from build123d import *
from build123d.topology import SkipClean

# Parameters (mm, degrees)
ESQUISSE1_R             = 1.2
BOSS_EXTRU_1_DEPTH      = 12
BOSS_EXTRU_2_DEPTH      = 12
ESQUISSE3_OUTSIDE_W     = 37.484
ESQUISSE3_OUTSIDE_H     = 73.419
ENL_V_MAT_EXTRU_1_DEPTH = 170.970209289
CONG_2_R                = 3
CONG_1_R                = 1.5
ESQUISSE7_W             = 0.946782305
ESQUISSE7_H             = 12
ENL_V_MAT_EXTRU_5_DEPTH = 15
CONG_3_R                = 1.5
ENL_V_MAT_EXTRU_3_DEPTH = 2
CONG_4_R                = 3


with BuildPart() as part:
    # Esquisse1 → Boss.-Extru.1 (new body)
    with BuildSketch(Plane(origin=(0, 0, 0), x_dir=(1, 0, 0), z_dir=(0, 1, 0))):
        with BuildLine():
            Line((5, -115), (5, -146))
            Line((5, -146), (-5, -146))
            Line((-5, -146), (-5, -115))
            ThreePointArc((-5, -115), (0, -110), (5, -115))
        make_face()
        with Locations(Location((0, -115, 0), (0, 0, 270))):
            Circle(ESQUISSE1_R, mode=Mode.SUBTRACT)
        with Locations(Location((0, -130, 0), (0, 0, 270))):
            Circle(ESQUISSE1_R, mode=Mode.SUBTRACT)
    extrude(amount=-BOSS_EXTRU_1_DEPTH)

    # Esquisse2 → Boss.-Extru.2 (add)
    with BuildSketch(Plane(origin=(0, 0, 0), x_dir=(1, 0, 0), z_dir=(0, 1, 0))):
        with BuildLine():
            ThreePointArc((2.297654972, -159.197635973), (2.500096708, -154.365285132), (2.549630638, -149.52894936))
            ThreePointArc((2.549630638, -149.52894936), (-1.115535331, -144.03526605), (-7.609239761, -145.237680564))
            ThreePointArc((-7.609239761, -145.237680564), (-10.72587755, -148.106981091), (-13.96441251, -150.837953067))
            ThreePointArc((-13.96441251, -150.837953067), (-12.257608054, -167.514829553), (2.297654972, -159.197635973))
        make_face()
        with BuildLine():
            ThreePointArc((-11.452932946, -153.951226328), (-8.081311937, -151.108026363), (-4.836597406, -148.1208133))
            ThreePointArc((-4.836597406, -148.1208133), (-2.672029263, -147.720008461), (-1.450307273, -149.551236231))
            ThreePointArc((-1.450307273, -149.551236231), (-1.498545632, -154.261076504), (-1.695692457, -158.967036072))
            ThreePointArc((-1.695692457, -158.967036072), (-10.428850272, -163.95735222), (-11.452932946, -153.951226328))
        make_face(mode=Mode.SUBTRACT)
    extrude(amount=-BOSS_EXTRU_2_DEPTH)

    # Esquisse3 outside → Enlèv. mat.-Extru.1 (cut, through all)
    with BuildSketch(Plane(origin=(0, 0, 0), x_dir=(1, 0, 0), z_dir=(0, 1, 0))):
        with Locations((-6.343, -139.3105)):
            Rectangle(ESQUISSE3_OUTSIDE_W, ESQUISSE3_OUTSIDE_H)
        with BuildLine():
            Line((-13, -140.030172342), (-13, -110))
            Line((-13, -110), (0, -110))
            Line((0, -110), (0, -153.030172342))
            ThreePointArc((0, -153.030172342), (-9.192388155, -149.222560498), (-13, -140.030172342))
        make_face(mode=Mode.SUBTRACT)
    extrude(amount=-ENL_V_MAT_EXTRU_1_DEPTH, mode=Mode.SUBTRACT)

    # Congé2
    cong_2_edges = [part.edges().sort_by_distance(p)[0] for p in [
        (-5, -6, 143.765970759),
        (-10.40524253, -6, 147.823177404),
    ]]
    fillet(cong_2_edges, radius=CONG_2_R)

    # Congé1
    cong_1_edges = [part.edges().sort_by_distance(p)[0] for p in [
        (-7.535402248, -6, 150.623458563),
    ]]
    fillet(cong_1_edges, radius=CONG_1_R)

    # Esquisse5 → Enlèvement de matière-Révolution1 (revolve, cut)
    with BuildSketch(Plane(origin=(0, 0, 0), x_dir=(0, 0, -1), z_dir=(1, 0, 0))):
        with BuildLine():
            Line((-146, -12), (-115, -12))
            Line((-115, -12), (-115, -7))
            Line((-115, -7), (-135, -7))
            ThreePointArc((-135, -7), (-141.041522987, -8.308649429), (-146, -12))
        make_face()
        with BuildLine():
            Line((-146, 0), (-160, 0))
            Line((-160, 0), (-160, -32.619012861))
            ThreePointArc((-160, -32.619012861), (-156.352146256, -14.870773511), (-146, 0))
        make_face()
    revolve(axis=Axis((0, 0, 115), (0, -1, 0)), mode=Mode.SUBTRACT)

    # Symétrie1: part across plane


with BuildPart() as part_1:
    with SkipClean():  # the faces are left unmerged after this step: merging them gives an invalid solid
        add(part.part)
        add(part.part.mirror(Plane(origin=(0, 0, 0), x_dir=(0, 0, 1), z_dir=(1, 0, 0))))

    # Esquisse7 → Enlèv. mat.-Extru.5 (cut)
    with SkipClean():  # the faces are left unmerged after this step: merging them gives an invalid solid
        with BuildSketch(Plane(origin=(5, 0, 0), x_dir=(0, 0, -1), z_dir=(1, 0, 0))):
            with Locations((-152.473391152, -6)):
                Rectangle(ESQUISSE7_W, ESQUISSE7_H)
        extrude(amount=-ENL_V_MAT_EXTRU_5_DEPTH, mode=Mode.SUBTRACT)


with BuildPart() as enl_v_mat_extru_5_kept_piece:
    # of the separate pieces the step leaves, the one the design keeps (enl_v_mat_extru_5_pieces_kept)
    add(part_1.part.solids().sort_by_distance((0, 0, 146))[0])

    # Congé3
    # the kernel refuses this fillet: 1.5 mm, written as the material it takes off along each edge
    with BuildSketch(Plane(origin=(-1.456795034, -15.771881232, 152), x_dir=(0.005830598143572619, 0, -0.9999830019181767), z_dir=(0, 1, 0))) as cong_3_piece_1:
        with BuildLine():
            CenterArc((1.508771432, -1.49998095), CONG_3_R, 90.288765492, 90.045305066)
            Line((0.008796929, -1.508726847), (0, 0))
            ThreePointArc((0, 0), (0.750605801, -0.001891496), (1.501211601, 0))
        make_face()
    extrude(amount=12.495782984, mode=Mode.SUBTRACT)
    with BuildSketch(Plane(origin=(1.456795034, -15.771881232, 152), x_dir=(-1, 0, 0), z_dir=(0, 1, 0))) as cong_3_piece_2:
        with BuildLine():
            CenterArc((1.508752493, -1.5), CONG_3_R, 90, 90.045305066)
            ThreePointArc((0.008752962, -1.501186084), (0.006267945, -0.750582013), (0, 0))
            Line((0, 0), (1.508752493, 0))
        make_face()
    extrude(amount=12.495782984, mode=Mode.SUBTRACT)

    # Esquisse6 → Enlèv. mat.-Extru.3 (cut)
    with BuildSketch(Plane.XZ.offset(7)):
        Polygon((2.75, 116.58771324), (0, 118.175426481), (-2.75, 116.58771324), (-2.75, 113.41228676), (0, 111.824573519), (2.75, 113.41228676), align=None)
        Polygon((2.75, 131.58771324), (0, 133.175426481), (-2.75, 131.58771324), (-2.75, 128.41228676), (0, 126.824573519), (2.75, 128.41228676), align=None)
    extrude(amount=-ENL_V_MAT_EXTRU_3_DEPTH, mode=Mode.SUBTRACT)

    # Congé4
    cong_4_edges = [enl_v_mat_extru_5_kept_piece.edges().sort_by_distance(p)[0] for p in [
        (-3.75326222, -12, 145.771951883),
        (0, 0, 146),
    ]]
    fillet(cong_4_edges, radius=CONG_4_R)


solid = enl_v_mat_extru_5_kept_piece.part
Can you work these out from the model? Positions are in its coordinate system, mm. A direction names the side the tool comes from. Give positions to 0.01 mm unless a question says otherwise; leave off trailing zeros. Loops run counter-clockwise (first coordinate to the right, second up) from the corner with the lowest first, then second, coordinate; pieces in that order, holes last. Notation, with made-up numbers: (-38, 24.25) - (10, 24.25) arc R22 ccw to (10, 60.25) - close; hole circle Ø1 at (36, 16). An arc over 180 degrees is marked (long way). Return JSON: item names as keys, results as strings.
1. I want a section at C-C on y = -3. Give the number of separate pieces and of enclosed holes in the cut face, and give its area (3 significant figures).
Output values:
{"separate pieces": "1", "enclosed holes": "2", "area": "389 mm²"}
2. We'd pull the mould along Z, two halves only. Please class faces 1 (the face through (-2.7, -6.8, 147.71)), 2 (the face through (1.36, -6.01, 112.61)), 3 (the face through (-5, -3, 129)): +Z half, -Z half, draft (parallel to the pull), parting line (faces both ways), or undercut.
Output values:
{"face 1": "+Z half", "face 2": "undercut", "face 3": "draft"}
3. I want a section at A-A on z = 130. Please give me the cut outline in (x, y), and give its area (3 significant figures).
Output values:
{"outline": "(-5, -7) - (-2.75, -7) - (-2.75, -5) - (-1.2, -5) - (-1.2, 0) - (-5, 0) - close; (1.2, -5) - (2.75, -5) - (2.75, -7) - (5, -7) - (5, 0) - (1.2, 0) - close", "area": "47.0 mm²"}
4. I'm going to push flat-ended pins straight in: pin 1 Ø4 at (x, z) = (6.5, 145) entering from +Y; pin 2 Ø2.5 at (y, z) = (-4, 123) entering from -X; pin 3 Ø1.6 at (y, z) = (-6, 130) entering from +X; pin 4 Ø4 at (x, z) = (0, 130) entering from -Y. Where does each tip first touch, or does it pass through?
Output values:
{"pin 1": "stops at y = 0", "pin 2": "stops at x = -5", "pin 3": "stops at x = 5", "pin 4": "stops at y = -5"}
5. If I drill on line 1 (X direction, y = -1.65, z = 115); line 2 (X direction, y = -8, z = 148.5); line 3 (X direction, y = -1, z = 138), over which ranges is the centre line in solid material (lowest first)?
Output values:
{"line 1": "x = -5 to -1.2, 1.2 to 5", "line 2": "x = -9.05 to -5.23, -1.76 to 1.76, 5.23 to 9.05", "line 3": "x = -5 to 5"}
6. I want a section at B-B on z = 113. Please give me the cut outline in (x, y).
Output values:
{"outline": "(-4.58, -7) - (-2.04, -7) - (-2.04, -5) - (2.04, -5) - (2.04, -7) - (4.58, -7) - (4.58, 0) - (-4.58, 0) - close"}
7. For faces 4 (the face through (0, -5, 113.6)), 5 (the face through (0.46, -2.46, 116.11)), which set-ups out of +Z, -Z, +X, -X, +Y, -Y let a thin tool reach every point of the face, with its end or its side?
Output values:
{"face 4": "-Y", "face 5": "+Y, -Y"}
